Geometry: final body of the model. Coordinates: model frame, mm. Give positions to 0.01 mm unless a question says otherwise; leave off trailing zeros. Write each loop counter-clockwise with the first axis right and the second up, starting at its lowest first coordinate (ties: lowest second). Pieces come first, ordered by that corner, then holes.
from build123d import *

# Parameters (mm, degrees)
BOSS_EXTRUDE3_DEPTH = 10


with BuildPart() as part:
    # Sketch1 → Boss-Extrude3 (new body)
    with BuildSketch(Plane.XY):
        with BuildLine():
            Line((61.719673081, 1004.040138522), (90.121595591, 1063.443540058))
            ThreePointArc((90.121595591, 1063.443540058), (101.806598129, 1080.290626418), (116.685466786, 1094.39675525))
            ThreePointArc((116.685466786, 1094.39675525), (139.054779467, 1117.668267819), (166.244818626, 1135.065141607))
            ThreePointArc((166.244818626, 1135.065141607), (203.849887916, 1144.889885631), (241.454957205, 1135.065141607))
            ThreePointArc((241.454957205, 1135.065141607), (265.935060661, 1103.204515558), (271.717774961, 1063.443540058))
            ThreePointArc((271.717774961, 1063.443540058), (264.746706267, 1020.532699182), (249.993176003, 979.639308419))
            Line((249.993176003, 979.639308419), (217.557058689, 927.454623329))
            ThreePointArc((217.557058689, 927.454623329), (196.913476553, 892.129764254), (178.225545137, 855.732451558))
            ThreePointArc((178.225545137, 855.732451558), (160.866603962, 806.767718632), (144.678077696, 757.403667679))
            ThreePointArc((144.678077696, 757.403667679), (126.716261258, 693.277809244), (96.398038564, 633.985668597))
            ThreePointArc((96.398038564, 633.985668597), (72.892497642, 594.596356166), (44.675436223, 558.432481475))
            ThreePointArc((44.675436223, 558.432481475), (6.069688965, 498.228600511), (-28.843305621, 435.810703931))
            Line((-28.843305621, 435.810703931), (-61.080316316, 376.666682759))
            ThreePointArc((-61.080316316, 376.666682759), (-146.105172251, 458.069534428), (-256.734722378, 498.278401925))
            ThreePointArc((-256.734722378, 498.278401925), (-185.027496066, 605.596315922), (-126.015280279, 720.385772571))
            ThreePointArc((-126.015280279, 720.385772571), (-92.438560876, 793.893867743), (-40.411397842, 855.732451558))
            ThreePointArc((-40.411397842, 855.732451558), (-4.339376244, 896.978618456), (24.369918596, 943.649952439))
            ThreePointArc((24.369918596, 943.649952439), (44.675436223, 972.836536947), (61.719673081, 1004.040138522))
        make_face()
    extrude(amount=BOSS_EXTRUDE3_DEPTH)


solid = part.part
Q1. Ray query, line 1 along X through (y, z) = (454, 6); line 2 along Y through (x, z) = (247, 9.5); line 3 along Y through (x, z) = (52, 3.75). Return the intervals inside material, ascending.
Filled sheet:
line 1: x = -139.75 to -19.18
line 2: y = 974.82 to 1130.34
line 3: y = 566.96 to 985.28
Q2. Section C-C on x = -213.5. Output: boundary loops of the cut face in (y, z).
Filled sheet:
outline: (488.67, 0) - (559.76, 0) - (559.76, 10) - (488.67, 10) - close
Q3. Section A-A on z = 4.25. Output: boundary loops of the cut face in (x, y), plus the area to 3 significant figures.
Filled sheet:
outline: (-256.73, 498.28) arc R285.67 cw to (-61.08, 376.67) - (-28.84, 435.81) arc R1187.96 cw to (44.68, 558.43) arc R368.49 ccw to (96.4, 633.99) arc R334.24 ccw to (144.68, 757.4) arc R2182.39 cw to (178.23, 855.73) arc R750.54 cw to (217.56, 927.45) - (249.99, 979.64) arc R235.08 ccw to (271.72, 1063.44) arc R79.53 ccw to (241.45, 1135.07) arc R76.88 ccw to (166.24, 1135.07) arc R137.11 ccw to (116.69, 1094.4) arc R99.88 ccw to (90.12, 1063.44) - (61.72, 1004.04) arc R329.67 cw to (24.37, 943.65) arc R328.29 cw to (-40.41, 855.73) arc R299.15 ccw to (-126.02, 720.39) arc R1130.92 cw to start
area: 156,000 mm2
Q4. Section B-B on y = 676.5. Output: boundary loops of the cut face in (x, z).
Filled sheet:
outline: (-146.63, 0) - (119.62, 0) - (119.62, 10) - (-146.63, 10) - close
Q5. Pin query (flat end, axial travel): P1, Ø1.5, axis at y = 889.5, z = 5.5, coming from the -X side; P2, Ø2, axis at x = -123, z = 4.5, coming from the -Y side; P3, Ø1.5, axis at x = -43, z = 6, coming from the +Y side. Return the tip coordinate at first contact, or that it passes through.
Filled sheet:
P1: stops at x = -10.6
P2: stops at y = 441.31
P3: stops at y = 854.05
